Autodesk Inventor part; units mm, degrees
ref_plane "YZ Plane" through (0, 0, 0) normal (1, 0, 0) x (0, 1, 0)
ref_plane "XZ Plane" through (0, 0, 0) normal (0, 1, 0) x (-1, 0, 0)
ref_plane "XY Plane" through (0, 0, 0) normal (0, 0, 1) x (1, 0, 0)
sketch "Sketch1" plane through (0, 0, 0) normal (0, 0, 1) x (1, 0, 0)
  line L0 (-28.6614, -59.685) -> (66.3386, -59.685)
  line L1 (66.3386, -59.685) -> (66.3386, 60.315)
  line L2 (66.3386, 60.315) -> (-28.6614, 60.315)
  line L3 (-28.6614, 60.315) -> (-28.6614, -59.685)
  point P0 (0, 0)
  dimension "d0" = 120
  dimension "d1" = 95
extrude "Extrusion1" add sketch "Sketch1" along normal blind 6
sketch "Sketch3" plane through (0, 0, 0) normal (0, 0, -1) x (-1, 0, 0)
  line L0 (-66.3386, 60.315) -> (28.6614, 60.315)
  line L1 (28.6614, 60.315) -> (28.6614, 53.315)
  line L2 (28.6614, 60.315) -> (28.6614, -59.685)
  line L3 (28.6614, 53.315) -> (-6.3386, 53.315)
  line L4 (-6.3386, 53.315) -> (-6.3386, -21.685)
  line L5 (-6.3386, -21.685) -> (28.6614, -21.685)
  line L6 (28.6614, -21.685) -> (28.6614, -59.685)
  line L7 (28.6614, -59.685) -> (-66.3386, -59.685)
  line L8 (28.6614, -59.685) -> (-66.3386, -59.685)
  line L9 (-66.3386, -59.685) -> (-66.3386, 60.315)
  line L10 (-66.3386, -59.685) -> (-66.3386, 60.315)
  line L11 (-66.3386, 60.315) -> (28.6614, 60.315)
  point P0 (0, 0)
  dimension "d9" = 7
  dimension "d10" = 35
  dimension "d11" = 75
extrude "Extrusion3" add sketch "Sketch3" along normal blind 3 contours L0 L1 L3 L4 L5 L2 L7 L9
fillet "Fillet1" radius 7 2 edges at (6.3386, -21.685, -1.5) (6.3386, 53.315, -1.5)
sketch "Sketch4" plane through (0, 0, 0) normal (0, 0, -1) x (-1, 0, 0)
  circle A0 centre (6.1614, 42.6422) radius 3.3
  circle A1 centre (21.1614, 42.6422) radius 3.3
  circle A2 centre (21.1614, -11.3578) radius 3.3
  circle A3 centre (6.1614, -11.3578) radius 3.3
  point P0 (0, 0)
extrude "Extrusion4" cut sketch "Sketch4" against normal through all
properties part number "Internal support motor-ball bracket"
Here's how the part is built. I have some questions about the finished solid (model axes, mm). A direction names the side the tool comes from. Coordinates: 2 decimals unless noted, no trailing zeros. Write each loop counter-clockwise with the first axis right and the second up, starting at its lowest first coordinate (ties: lowest second). Pieces come first, ordered by that corner, then holes.
Item 1: I want a section at C-C on y = 30. Write out the boundary of the cut face in (x, z), and give its area (3 significant figures).
Item 2: If I drill on line 1 (Y direction, x = -6.5, z = 3) (3 decimals); line 2 (X direction, y = -12, z = 2.75); line 3 (Z direction, x = 1, y = 42), over which ranges is the centre line in solid material (lowest first)?
Item 3: I want a section at B-B on z = -1.25. Write out the boundary of the cut face in (x, y) (3 decimals), and give its area (3 significant figures).
Item 4: I want a section at D-D on y = -16.5. Write out the boundary of the cut face in (x, z).
Item 5: Will these pins go through, and if not, where does the flat tip stop? pin 1 (17.5 mm diameter, centred on x = -2.5, y = 21.5, fed in from -Z); pin 2 (0.9 mm diameter, centred on y = 18.5, z = -1, fed in from -X); pin 3 (4 mm diameter, centred on x = -6.16, y = 42.64, fed in from -Z).
Item 6: On a 3-axis mill with a long thin cutter (end or side, diameter ignored), from which of +Z, -Z, +X, -X, +Y, -Y can I reach the whole of each face in a straight line? I mean faces 1 (the flat face through (20, 60.315, 1)), 2 (the flat face through (6.339, 16, -1)). Say none if no direction works.
Item 7: I want a section at A-A on x = -6. Write out the boundary of the cut face in (y, z) (3 decimals).
Findings below:
1. outline: (-28.66, 0) - (6.34, 0) - (6.34, -3) - (66.34, -3) - (66.34, 6) - (-28.66, 6) - close
1. area: 750 mm2
2. line 1: y = -59.685 to -14.64, -8.075 to 39.36, 45.925 to 60.315
2. line 2: x = -28.66 to -24.4, -17.92 to -9.4, -2.92 to 66.34
2. line 3: z = 0 to 6
3. outline: (-28.661, -59.685) - (66.339, -59.685) - (66.339, 60.315) - (-28.661, 60.315) - (-28.661, 53.315) - (-0.661, 53.315) arc R7 cw to (6.339, 46.315) - (6.339, -14.685) arc R7 cw to (-0.661, -21.685) - (-28.661, -21.685) - close
3. area: 8,800 mm2
4. outline: (-28.66, 0) - (6.1, 0) - (6.1, -3) - (66.34, -3) - (66.34, 6) - (-28.66, 6) - close
5. pin 1: stops at z = 0
5. pin 2: stops at x = 6.34
5. pin 3: passes through
6. face 1: +Z, -Z, +X, -X, +Y
6. face 2: -Z, -X
7. outline: (-59.685, -3) - (-21.685, -3) - (-21.685, 0) - (-14.654, 0) - (-14.654, 6) - (-59.685, 6) - close; (-8.062, 0) - (39.346, 0) - (39.346, 6) - (-8.062, 6) - close; (45.938, 0) - (53.315, 0) - (53.315, -3) - (60.315, -3) - (60.315, 6) - (45.938, 6) - close
